Input: part model. Units: mm. Frame: model coordinates. A direction names the side the tool comes from. Round coordinates to 2 decimals unless told otherwise and drop trailing zeros. Order: outer loops, then holes, each group sorted by start corner. A loop starts at its lowest first (then second) coordinate and runs counter-clockwise, first axis right, second up. Notation, with made-up numbers: (57, -6) -> (77, -6) arc R21 cw to (77, -2) -> close; hole circle Ø9 at (3.5, 29.5). An arc over 180 degrees is marked (long way). Use a Markdown table: item, result.
from build123d import *

# Parameters (mm, degrees)
EXTRUDE_1_DEPTH     = 4
CUT_EXTRUDE_1_REACH = 61.822
SKETCH_2_R          = 2.1
FILLET_1_R          = 2


with BuildPart() as part:
    # 草图1 → 凸台-拉伸1 (new body)
    with BuildSketch(Plane.XY):
        with BuildLine():
            Line((18.657436361, 56), (-20, 56))
            Line((-20, 56), (-20, 21))
            Line((-20, 21), (-20, -21))
            Line((-20, -21), (20, -21))
            Line((20, -21), (20, 21))
            Line((20, 21), (2.525225805, 31))
            Line((2.525225805, 31), (2.525225805, 46))
            Line((2.525225805, 46), (19.341476647, 52.120614758))
            ThreePointArc((19.341476647, 52.120614758), (20.627051867, 54.347296355), (18.657436361, 56))
        make_face()
    extrude(amount=EXTRUDE_1_DEPTH)

    # 草图2 → 切除-拉伸1 (cut, up to next)
    with BuildSketch(Plane.XY.offset(4), mode=Mode.PRIVATE) as cut_extrude_1_sk1:
        with Locations((-10, -15.5)):
            Circle(SKETCH_2_R)
    cut_extrude_1_tool1 = extrude(cut_extrude_1_sk1.sketch, amount=-CUT_EXTRUDE_1_REACH, mode=Mode.PRIVATE) & part.part
    # 草图2 → 切除-拉伸1 (cut, up to next)
    with BuildSketch(Plane.XY.offset(4), mode=Mode.PRIVATE) as cut_extrude_1_sk2:
        with Locations((-10, -1.5)):
            Circle(SKETCH_2_R)
    cut_extrude_1_tool2 = extrude(cut_extrude_1_sk2.sketch, amount=-CUT_EXTRUDE_1_REACH, mode=Mode.PRIVATE) & part.part
    # 草图2 → 切除-拉伸1 (cut, up to next)
    with BuildSketch(Plane.XY.offset(4), mode=Mode.PRIVATE) as cut_extrude_1_sk3:
        with Locations((10, -1.5)):
            Circle(SKETCH_2_R)
    cut_extrude_1_tool3 = extrude(cut_extrude_1_sk3.sketch, amount=-CUT_EXTRUDE_1_REACH, mode=Mode.PRIVATE) & part.part
    # 草图2 → 切除-拉伸1 (cut, up to next)
    with BuildSketch(Plane.XY.offset(4), mode=Mode.PRIVATE) as cut_extrude_1_sk4:
        with Locations((10, -15.5)):
            Circle(SKETCH_2_R)
    cut_extrude_1_tool4 = extrude(cut_extrude_1_sk4.sketch, amount=-CUT_EXTRUDE_1_REACH, mode=Mode.PRIVATE) & part.part
    add(cut_extrude_1_tool1.solids().sort_by_distance((-10, -15.5, 4))[0], mode=Mode.SUBTRACT)
    add(cut_extrude_1_tool2.solids().sort_by_distance((-10, -1.5, 4))[0], mode=Mode.SUBTRACT)
    add(cut_extrude_1_tool3.solids().sort_by_distance((10, -1.5, 4))[0], mode=Mode.SUBTRACT)
    add(cut_extrude_1_tool4.solids().sort_by_distance((10, -15.5, 4))[0], mode=Mode.SUBTRACT)

    # 圆角1
    fillet_1_edges = [part.edges().sort_by_distance(p)[0] for p in [
        (2.525225805, 46, 2),
        (2.525225805, 31, 2),
        (20, 21, 2),
        (20, -21, 2),
        (-20, -21, 2),
        (-20, 56, 2),
    ]]
    fillet(fillet_1_edges, radius=FILLET_1_R)


solid = part.part
1) Cut plane B-B on y = -1.5. Return loops of the section in (x, z), and give its area (3 significant figures).
Answer key:
| item | result |
|---|---|
| outline | (-20, 0) -> (-12.1, 0) -> (-12.1, 4) -> (-20, 4) -> close; (-7.9, 0) -> (7.9, 0) -> (7.9, 4) -> (-7.9, 4) -> close; (12.1, 0) -> (20, 0) -> (20, 4) -> (12.1, 4) -> close |
| area | 126 mm^2 |
2) Set-up query: faces 1 (the face through (7.9, -15.41, 2.03)), 2 (the face through (20, 0, 2)), 3 (the face through (2.788, 31.169, 2.028)). Return all of +Z, -Z, +X, -X, +Y, -Y with unobstructed straight access to the full face (end or side cutting, diameter ignored); none if empty.
Answer key:
| item | result |
|---|---|
| face 1 | +Z, -Z |
| face 2 | +Z, -Z, +X, -Y |
| face 3 | +Z, -Z, +X |
3) Cut plane D-D on x = 10. Return loops of the section in (y, z).
Answer key:
| item | result |
|---|---|
| outline | (-21, 0) -> (-17.6, 0) -> (-17.6, 4) -> (-21, 4) -> close; (-13.4, 0) -> (-3.6, 0) -> (-3.6, 4) -> (-13.4, 4) -> close; (0.6, 0) -> (26.72, 0) -> (26.72, 4) -> (0.6, 4) -> close; (48.72, 0) -> (56, 0) -> (56, 4) -> (48.72, 4) -> close |
4) Contact query for flat-ended pins moving along their axis: P1, Ø6.5, axis at x = -10, y = -1.5, coming from the -Z side; P2, Ø1.2, axis at y = -1.5, z = 1, coming from the +X side; P3, Ø4, axis at x = -10, y = -15.5, coming from the -Z side. Output: stop coordinate, or through.
Answer key:
| item | result |
|---|---|
| P1 | stops at z = 0 |
| P2 | stops at x = 20 |
| P3 | passes through |
5) Cut plane C-C on z = 3.35. Return loops of the section in (x, y).
Answer key:
| item | result |
|---|---|
| outline | (-20, -19) arc R2 ccw to (-18, -21) -> (18, -21) arc R2 ccw to (20, -19) -> (20, 19.84) arc R2 ccw to (18.99, 21.58) -> (3.53, 30.42) arc R2 cw to (2.53, 32.16) -> (2.53, 44.6) arc R2 cw to (3.84, 46.48) -> (19.34, 52.12) arc R2 ccw to (18.66, 56) -> (-18, 56) arc R2 ccw to (-20, 54) -> close; hole circle Ø4.2 at (-10, -15.5); hole circle Ø4.2 at (-10, -1.5); hole circle Ø4.2 at (10, -15.5); hole circle Ø4.2 at (10, -1.5) |
6) Cut plane A-A on x = -10. Return loops of the section in (y, z), and give its area (3 significant figures).
Answer key:
| item | result |
|---|---|
| outline | (-21, 0) -> (-17.6, 0) -> (-17.6, 4) -> (-21, 4) -> close; (-13.4, 0) -> (-3.6, 0) -> (-3.6, 4) -> (-13.4, 4) -> close; (0.6, 0) -> (56, 0) -> (56, 4) -> (0.6, 4) -> close |
| area | 274 mm^2 |
7) Draft query along X for faces 4 (the face through (11.37, 25.94, 1.97)), 5 (the face through (0, -21, 2)), 6 (the face through (-12.1, -15.41, 2.03)). Return one class per face: released by +X, released by -X, zero draft, split by the parting line, or undercut.
Answer key:
| item | result |
|---|---|
| face 4 | released by +X |
| face 5 | zero draft |
| face 6 | undercut |
8) Ray query, probe 1 along Y at (x, z) = (-10, 2.65); probe 2 along Y at (x, z) = (10, 1.25); probe 3 along Y at (x, z) = (11.5, 2.5). Return the intervals inside material, ascending.
Answer key:
| item | result |
|---|---|
| probe 1 | y = -21 to -17.6, -13.4 to -3.6, 0.6 to 56 |
| probe 2 | y = -21 to -17.6, -13.4 to -3.6, 0.6 to 26.72, 48.72 to 56 |
| probe 3 | y = -21 to -16.97, -14.03 to -2.97, -0.03 to 25.86, 49.27 to 56 |
